Could you check a few things on this model? Use its own coordinates, in mm. A direction names the side the tool comes from. Give positions to 0.01 mm unless a question says otherwise; leave off trailing zeros. Write each loop counter-clockwise with the first axis right and the second up, starting at its lowest first coordinate (ties: lowest second). Pieces come first, ordered by that corner, then holes. Notation, with made-up numbers: (35, 15.5) - (53, 15.5) arc R8 cw to (53, 22.5) - close; hole circle Ø1 at (-19.75, 59.5). An arc over 180 degrees is marked (long way). Answer in a Markdown table with one row per item.
from build123d import *

# Parameters (mm, degrees)
SKETCH1_R                                      = 27.5
BOSS_EXTRUDE1_DEPTH                            = 8
M4_CLEARANCE_HOLE1_D                           = 4.5
CIRPATTERN1_COUNT                              = 4
SKETCH11_R                                     = 6
CUT_EXTRUDE1_DEPTH                             = 143.673807756
CSK_FOR_6_FLAT_HEAD_MACHINE_SCREW1_D           = 4.064
CSK_FOR_6_FLAT_HEAD_MACHINE_SCREW1_CSINK_D     = 7.366
CSK_FOR_6_FLAT_HEAD_MACHINE_SCREW1_CSINK_ANGLE = 82
CIRPATTERN2_COUNT                              = 6


with BuildPart() as part:
    # Sketch1 → Boss-Extrude1 (new body)
    with BuildSketch(Plane(origin=(0, 0, 0), x_dir=(1, 0, 0), z_dir=(0, 1, 0))):
        with Locations(Location((0, 0, 0), (0, 0, 270))):
            Circle(SKETCH1_R)
    extrude(amount=BOSS_EXTRUDE1_DEPTH)

    # M4 Clearance Hole1 (through all)
    with Locations(Plane(origin=(0, 8, 0), x_dir=(1, 0, 0), z_dir=(0, 1, 0))):
        with Locations((0, 15)):
            m4_clearance_hole1 = Hole(M4_CLEARANCE_HOLE1_D / 2)

    # CirPattern1: M4 Clearance Hole1 ×4 about axis
    cirpattern1_axis = Axis((0, 0, 0), (0, 1, 0))
    for i in range(1, CIRPATTERN1_COUNT):
        add(m4_clearance_hole1.rotate(cirpattern1_axis, i * 360 / CIRPATTERN1_COUNT), mode=Mode.SUBTRACT)

    # Sketch6 → Revolve1 (revolve)
    with BuildSketch(Plane.XY, mode=Mode.PRIVATE) as revolve1_sk:
        Polygon((76.92225691, 52.5), (27.5, 8), (17.5, 8), (17.5, 0), (27.5, 0), (85.807157029, 52.5), align=None)
        Polygon((85.807157029, 52.5), (78.032869425, 45.5), (93.807157029, 45.5), (93.807157029, 52.5), align=None)
    revolve(revolve1_sk.sketch.rotate(Axis((0, 8, 0), (0, -1, 0)), 90), axis=Axis((0, 8, 0), (0, -1, 0)))

    # Sketch11 → Cut-Extrude1 (cut, through all)
    with BuildSketch(Plane.XZ):
        with Locations(Location((0, 0, 0), (0, 0, 270))):
            Circle(SKETCH11_R)
    extrude(amount=-CUT_EXTRUDE1_DEPTH, mode=Mode.SUBTRACT)

    # CSK for #6 Flat Head Machine Screw1 (through all)
    with Locations(Plane.XZ.offset(-45.5)):
        with Locations((85.5, 0)):
            csk_for_6_flat_head_machine_screw1 = CounterSinkHole(CSK_FOR_6_FLAT_HEAD_MACHINE_SCREW1_D / 2, CSK_FOR_6_FLAT_HEAD_MACHINE_SCREW1_CSINK_D / 2, counter_sink_angle=CSK_FOR_6_FLAT_HEAD_MACHINE_SCREW1_CSINK_ANGLE)

    # CirPattern2: CSK for #6 Flat Head Machine Screw1 ×6 about axis
    cirpattern2_axis = Axis((0, 0, 0), (0, 1, 0))
    for i in range(1, CIRPATTERN2_COUNT):
        add(csk_for_6_flat_head_machine_screw1.rotate(cirpattern2_axis, i * 360 / CIRPATTERN2_COUNT), mode=Mode.SUBTRACT)

    # Split1
    split(bisect_by=Plane(origin=(60, 0, 0), x_dir=(0, 0, 1), z_dir=(1, 0, 0)), keep=Keep.BOTTOM)


solid = part.part
1) Imagine slicing it at C-C (z = 0). List the corners of the cut face in (x, y) for me, then the cut area to 3 significant figures.
Check values:
| item | result |
|---|---|
| outline | (-93.81, 45.5) - (-89.18, 45.5) - (-87.53, 47.4) - (-87.53, 52.5) - (-93.81, 52.5) - close; (-83.47, 47.4) - (-81.82, 45.5) - (-78.03, 45.5) - (-27.5, 0) - (-17.25, 0) - (-17.25, 8) - (-27.5, 8) - (-76.92, 52.5) - (-83.47, 52.5) - close; (-12.75, 0) - (-6, 0) - (-6, 8) - (-12.75, 8) - close; (6, 0) - (12.75, 0) - (12.75, 8) - (6, 8) - close; (17.25, 0) - (27.5, 0) - (60, 29.26) - (60, 37.26) - (27.5, 8) - (17.25, 8) - close |
| area | 1,010 mm2 |
2) Will these pins go through, and if not, where does the flat tip stop? P1, Ø4, axis at x = -31.5, z = -8.5, coming from the -Y side; P2, Ø2.5, axis at x = -85.5, z = 0, coming from the +Y side; P3, Ø3, axis at x = -40, z = -38.5, coming from the -Y side; P4, Ø3, axis at x = -55.5, z = -47, coming from the +Y side.
Check values:
| item | result |
|---|---|
| P1 | stops at y = 2.82 |
| P2 | passes through |
| P3 | stops at y = 23.88 |
| P4 | stops at y = 50.07 |
3) Imagine slicing it at D-D (y = 15.5). List the corners of the cut face in (x, z) for me, then the cut area to 3 significant figures.
Check values:
| item | result |
|---|---|
| outline | circle Ø89.43 at (0, 0); hole circle Ø71.66 at (0, 0) |
| area | 2,250 mm2 |
4) Imagine slicing it at B-B (x = -85.5). List the corners of the cut face in (y, z) for me.
Check values:
| item | result |
|---|---|
| outline | (45.5, -38.59) - (52.5, -38.59) - (52.5, -2.03) - (47.4, -2.03) - (45.5, -3.68) - close; (45.5, 3.68) - (47.4, 2.03) - (52.5, 2.03) - (52.5, 38.59) - (45.5, 38.59) - close |
5) On a 3-axis mill with a long thin cutter (end or side, diameter ignored), from which of +Z, -Z, +X, -X, +Y, -Y can I reach the whole of each face in a straight line? I mean faces 1 (the face through (6.5, 8, -0.4)), 2 (the face through (42.31, 49.99, 76.03)), 3 (the face through (-80, 45.5, 0)). Say none if no direction works.
Check values:
| item | result |
|---|---|
| face 1 | +Y |
| face 2 | +Y, -Y |
| face 3 | -Y |
6) Imagine slicing it at A-A (x = 0). List the corners of the cut face in (y, z) for me, then the cut area to 3 significant figures.
Check values:
| item | result |
|---|---|
| outline | (0, -27.5) - (45.5, -78.03) - (45.5, -93.81) - (52.5, -93.81) - (52.5, -76.92) - (8, -27.5) - (8, -17.25) - (0, -17.25) - close; (0, -12.75) - (8, -12.75) - (8, -6) - (0, -6) - close; (0, 6) - (8, 6) - (8, 12.75) - (0, 12.75) - close; (0, 17.25) - (8, 17.25) - (8, 27.5) - (52.5, 76.92) - (52.5, 93.81) - (45.5, 93.81) - (45.5, 78.03) - (0, 27.5) - close |
| area | 1,300 mm2 |
7) If I drill on line 1 (Z direction, x = 42.75, y = 51); line 2 (Y direction, x = -21, z = 85); line 3 (X direction, y = 5.75, z = 0), over which ranges is the centre line in solid material (lowest first)?
Check values:
| item | result |
|---|---|
| line 1 | z = -83.5 to -76.08, -72.01 to -61.94, 61.94 to 72.01, 76.08 to 83.5 |
| line 2 | y = 45.5 to 52.5 |
| line 3 | x = -33.89 to -17.25, -12.75 to -6, 6 to 12.75, 17.25 to 33.89 |
